Source: CAD feature listing. Evaluate the final solid. Frame: model axes, mm. A direction names the side the tool comes from. Coordinates: 2 decimals unless noted, no trailing zeros. Write each loop counter-clockwise with the first axis right and the second up, starting at its lowest first coordinate (ties: lowest second). Pieces come first, ordered by that corner, then holes. Notation, with made-up numbers: M 6.25,-27.75 L 46.25,-27.75 A20 ccw 46.25,-9.75 Z; hole C -10.5,1.5 d11. An arc over 180 degrees is marked long. Write item = value, one per line. Start each with the question number.
1. Section query B-B (y = 0.95). Give the number of separate pieces and of enclosed holes in the cut face, then the cut area to 3 significant figures.
2. Section query A-A (z = -290). Output: boundary loops of the cut face in (x, y).
3. Access query for faces 4 (the face through (210, 2, -40)), 5 (the face through (184.758, 1.972, -148.505)). Directions: +Z, -Z, +X, -X, +Y, -Y. A direction counts if a zero-diameter tool reaches every point of the face in a straight line with its end or side. Return the directions, or none.
4. Pin query (flat end, axial travel): pin 1 Ø3.5 at (x, z) = (-150, -310) entering from -Y; pin 2 Ø1.2 at (y, z) = (2, -251.5) entering from +X; pin 3 Ø5 at (x, z) = (-20, -310) entering from +Y. Return the tip coordinate at first contact, or that it passes through.
5. Line query: line 1 along Z through (x, y) = (18.5, 3.45); line 2 along Z through (x, y) = (250, 0.9); line 3 along X through (y, z) = (3.15, -271). Output: solid intervals per line, ascending.
6. Pull-direction query (Z, two-part tool) for faces 1 (the face through (-24, 4, -151)), 2 (the face through (-210, 2, -40)), 3 (the face through (-180.72, 1.97, -320.49)); classes: pulls with the +Z half, pulls with the -Z half, needs draft (parallel to the pull), parting line crosses it, or undercut.
```python
from build123d import *

# Parameters (mm, degrees)
SKETCH1_R           = 4.5
SKETCH1_R_2         = 2
SKETCH1_R_3         = 5.5
BOSS_EXTRUDE1_DEPTH = 4


with BuildPart() as part:
    # Sketch1 → Boss-Extrude1 (new body)
    with BuildSketch(Plane(origin=(0, 0, 0), x_dir=(1, 0, 0), z_dir=(0, 1, 0))):
        with BuildLine():
            Line((-270, 15), (-235, 15))
            Line((-235, 15), (-185, 65))
            Line((-185, 65), (-185, 142))
            ThreePointArc((-185, 142), (-197, 154), (-185, 166))
            Line((-185, 166), (-185, 310))
            ThreePointArc((-185, 310), (-180.606601718, 320.606601718), (-170, 325))
            Line((-170, 325), (170, 325))
            ThreePointArc((170, 325), (180.606601718, 320.606601718), (185, 310))
            Line((185, 310), (185, 166))
            ThreePointArc((185, 166), (197, 154), (185, 142))
            Line((185, 142), (185, 65))
            Line((185, 65), (235, 15))
            Line((235, 15), (270, 15))
            ThreePointArc((270, 15), (285, 0), (270, -15))
            Line((270, -15), (-270, -15))
            ThreePointArc((-270, -15), (-285, 0), (-270, 15))
        make_face()
        with Locations(Location((-170, 310, 0), (0, 0, 270))):
            Circle(SKETCH1_R, mode=Mode.SUBTRACT)
        with Locations(Location((170, 310, 0), (0, 0, 270))):
            Circle(SKETCH1_R, mode=Mode.SUBTRACT)
        with Locations(Location((-270, 0, 0), (0, 0, 270))):
            Circle(SKETCH1_R, mode=Mode.SUBTRACT)
        with Locations(Location((270, 0, 0), (0, 0, 270))):
            Circle(SKETCH1_R, mode=Mode.SUBTRACT)
        with Locations(Location((0, 310, 0), (0, 0, 270))):
            Circle(SKETCH1_R_2, mode=Mode.SUBTRACT)
        with Locations(Location((-150, 310, 0), (0, 0, 270))):
            Circle(SKETCH1_R_2, mode=Mode.SUBTRACT)
        with Locations(Location((150, 310, 0), (0, 0, 270))):
            Circle(SKETCH1_R_2, mode=Mode.SUBTRACT)
        with Locations(Location((0, 0, 0), (0, 0, 270))):
            Circle(SKETCH1_R_2, mode=Mode.SUBTRACT)
        with Locations(Location((-150, 0, 0), (0, 0, 270))):
            Circle(SKETCH1_R_2, mode=Mode.SUBTRACT)
        with Locations(Location((150, 0, 0), (0, 0, 270))):
            Circle(SKETCH1_R_2, mode=Mode.SUBTRACT)
        with Locations(Location((-185, 154, 0), (0, 0, 270))):
            Circle(SKETCH1_R_3, mode=Mode.SUBTRACT)
        with Locations(Location((-185, 162, 0), (0, 0, 270))):
            Circle(SKETCH1_R_2, mode=Mode.SUBTRACT)
        with Locations(Location((-177, 154, 0), (0, 0, 270))):
            Circle(SKETCH1_R_2, mode=Mode.SUBTRACT)
        with Locations(Location((-185, 146, 0), (0, 0, 270))):
            Circle(SKETCH1_R_2, mode=Mode.SUBTRACT)
        with Locations(Location((-193, 154, 0), (0, 0, 270))):
            Circle(SKETCH1_R_2, mode=Mode.SUBTRACT)
        with Locations(Location((185, 162, 0), (0, 0, 90))):
            Circle(SKETCH1_R_2, mode=Mode.SUBTRACT)
        with Locations(Location((177, 154, 0), (0, 0, 90))):
            Circle(SKETCH1_R_2, mode=Mode.SUBTRACT)
        with Locations(Location((185, 146, 0), (0, 0, 90))):
            Circle(SKETCH1_R_2, mode=Mode.SUBTRACT)
        with Locations(Location((193, 154, 0), (0, 0, 90))):
            Circle(SKETCH1_R_2, mode=Mode.SUBTRACT)
        with Locations(Location((185, 154, 0), (0, 0, 90))):
            Circle(SKETCH1_R_3, mode=Mode.SUBTRACT)
        with Locations(Location((-130, 310, 0), (0, 0, 270))):
            Circle(SKETCH1_R_2, mode=Mode.SUBTRACT)
        with Locations(Location((130, 310, 0), (0, 0, 270))):
            Circle(SKETCH1_R_2, mode=Mode.SUBTRACT)
        with Locations(Location((-20, 310, 0), (0, 0, 270))):
            Circle(SKETCH1_R_2, mode=Mode.SUBTRACT)
        with Locations(Location((20, 310, 0), (0, 0, 270))):
            Circle(SKETCH1_R_2, mode=Mode.SUBTRACT)
        with Locations(Location((-250, 0, 0), (0, 0, 270))):
            Circle(SKETCH1_R_2, mode=Mode.SUBTRACT)
        with Locations(Location((-230, 0, 0), (0, 0, 270))):
            Circle(SKETCH1_R_2, mode=Mode.SUBTRACT)
        with Locations(Location((-20, 0, 0), (0, 0, 270))):
            Circle(SKETCH1_R_2, mode=Mode.SUBTRACT)
        with Locations(Location((20, 0, 0), (0, 0, 90))):
            Circle(SKETCH1_R_2, mode=Mode.SUBTRACT)
        with Locations(Location((230, 0, 0), (0, 0, 90))):
            Circle(SKETCH1_R_2, mode=Mode.SUBTRACT)
        with Locations(Location((250, 0, 0), (0, 0, 90))):
            Circle(SKETCH1_R_2, mode=Mode.SUBTRACT)
    extrude(amount=BOSS_EXTRUDE1_DEPTH)

    # Chamfer1
    # the kernel refuses this chamfer: 10 mm, written as the material it adds along each edge
    with BuildSketch(Plane(origin=(-185, 0, -142), x_dir=(0.026309669702560337, 0, 0.99965384072695), z_dir=(0, 1, 0))) as chamfer1_piece_1:
        with BuildLine():
            Line((7.93978752, 0), (-1.800869825, -5.618003075))
            Line((-1.800869825, -5.618003075), (-1.976561079, -5.522438525))
            ThreePointArc((-1.976561079, -5.522438525), (-0.637668429, -2.883002495), (-0.199930768, 0.005261934))
            Line((-0.199930768, 0.005261934), (0.005261934, 0.199930768))
            ThreePointArc((0.005261934, 0.199930768), (3.972407738, 0.09552033), (7.945049453, 0.199930768))
            Line((7.945049453, 0.199930768), (7.93978752, 0))
        make_face()
    extrude(amount=4)
    with BuildSketch(Plane(origin=(-185, 0, -166), x_dir=(-0.9599725502617332, 0, 0.2800940962319344), z_dir=(0, 1, 0))) as chamfer1_piece_2:
        with BuildLine():
            Line((5.899583941, 0), (-2.423649516, -7.560829907))
            Line((-2.423649516, -7.560829907), (-2.615644026, -7.504811088))
            ThreePointArc((-2.615644026, -7.504811088), (-1.303553405, -3.753651008), (-0.19199451, 0.056018819))
            Line((-0.19199451, 0.056018819), (0.056018819, 0.19199451))
            ThreePointArc((0.056018819, 0.19199451), (2.9400505, -0.272813985), (5.862210991, 0.19647713))
            Line((5.862210991, 0.19647713), (5.899583941, 0))
        make_face()
    extrude(amount=4)

    # Chamfer2
    # the kernel refuses this chamfer: 10 mm, written as the material it adds along each edge
    with BuildSketch(Plane(origin=(185, 0, -166), x_dir=(0.9599725502617332, 0, 0.2800940962319344), z_dir=(0, 1, 0))) as chamfer2_piece_1:
        with BuildLine():
            Line((5.899583941, 0), (-2.423649516, 7.560829907))
            Line((-2.423649516, 7.560829907), (-2.615644026, 7.504811088))
            ThreePointArc((-2.615644026, 7.504811088), (-1.303553405, 3.753651008), (-0.19199451, -0.056018819))
            Line((-0.19199451, -0.056018819), (0.056018819, -0.19199451))
            ThreePointArc((0.056018819, -0.19199451), (2.9400505, 0.272813985), (5.862210991, -0.19647713))
            Line((5.862210991, -0.19647713), (5.899583941, 0))
        make_face()
    extrude(amount=4)
    with BuildSketch(Plane(origin=(185, 0, -142), x_dir=(-0.026309669702560337, 0, 0.99965384072695), z_dir=(0, 1, 0))) as chamfer2_piece_2:
        with BuildLine():
            Line((7.93978752, 0), (-1.800869825, 5.618003075))
            Line((-1.800869825, 5.618003075), (-1.976561079, 5.522438525))
            ThreePointArc((-1.976561079, 5.522438525), (-0.637668429, 2.883002495), (-0.199930768, -0.005261934))
            Line((-0.199930768, -0.005261934), (0.005261934, -0.199930768))
            ThreePointArc((0.005261934, -0.199930768), (3.972407738, -0.09552033), (7.945049453, -0.199930768))
            Line((7.945049453, -0.199930768), (7.93978752, 0))
        make_face()
    extrude(amount=4)


solid = part.part
```
Results are:
q1.separate_pieces = 1
q1.enclosed_holes = 30
q1.area = 134,000 mm^2
q2.outline = M -185,0 L 185,0 L 185,4 L -185,4 Z
q3.face_4 = +X, +Y, -Y
q3.face_5 = +Y, -Y
q4.pin_1 = through
q4.pin_2 = 185
q4.pin_3 = 4
q5.line_1 = -325 to -311.32, -308.68 to -1.32, 1.32 to 15
q5.line_2 = -15 to -2, 2 to 15
q5.line_3 = -185 to 185
q6.face_1 = needs draft
q6.face_2 = undercut
q6.face_3 = pulls with the -Z half
